Autodesk Inventor part; units mm, degrees
ref_plane "YZ Plane" through (0, 0, 0) normal (1, 0, 0) x (0, 1, 0)
ref_plane "XZ Plane" through (0, 0, 0) normal (0, 1, 0) x (-1, 0, 0)
ref_plane "XY Plane" through (0, 0, 0) normal (0, 0, 1) x (1, 0, 0)
sketch "Sketch1" plane through (0, 0, 0) normal (0, 1, 0) x (-1, 0, 0)
  circle A0 centre (0, 0) radius 30
  dimension "d0" = 60
extrude "Extrusion1" add sketch "Sketch1" along normal blind 10
sketch "Sketch2" plane through (0, 10, 0) normal (0, 1, 0) x (1, 0, 0)
  circle A0 centre (0, 0) radius 5
  dimension "d3" = 10
extrude "Extrusion2" cut sketch "Sketch2" against normal through all
sketch "Sketch3" plane through (0, 10, 0) normal (0, 1, 0) x (1, 0, 0)
  circle A0 centre (0, 0) radius 25
  dimension "d6" = 50
extrude "Extrusion3" add sketch "Sketch3" along normal blind 20
sketch "Sketch5" plane through (0, 30, 0) normal (0, 1, 0) x (1, 0, 0)
  circle A0 centre (0, 0) radius 30
  dimension "d9" = 60
extrude "Extrusion4" add sketch "Sketch5" along normal blind 10
sketch "Sketch6" plane through (0, 40, 0) normal (0, 1, 0) x (1, 0, 0)
  circle A0 centre (0, 0) radius 5
  dimension "d12" = 10
extrude "Extrusion5" cut sketch "Sketch6" against normal through all
properties part number "pulley"
Check sheet for the modelled part. Datum: model origin and axes. Units: mm. A direction names the side the tool comes from. Give positions to 0.01 mm unless a question says otherwise; leave off trailing zeros. Loops run counter-clockwise (first coordinate to the right, second up) from the corner with the lowest first, then second, coordinate; pieces in that order, holes last. Notation, with made-up numbers: M 78,29 L 135,29 A21 cw 135,53 Z; hole C 51.5,59 d3. An arc over 180 degrees is marked long. Use a Markdown table: item, result. Add a question column.
Q1. Scan lines: line 1 along Z through (x, y) = (0, 24); line 2 along Y through (x, z) = (10.5, 26). Record each from-to range of solid material in increasing order. Write a range as [from, to].
Q2. Sectioned sample at A-A, the plane x = 0. Record the cut outline in (y, z), then the cut area to 3 significant figures.
Q3. Mould release check, pull along Y, two halves, no side actions. Record for faces 3 (the cylindrical face through (23.846, 19.86, 7.509)), 4 (the flat face through (0, 40, 6)), 5 (the flat face through (0, 0, -6)), 6 (the cylindrical face through (-29.97, 34.93, 1.32)): pulls with the +Y half, pulls with the -Y half, needs draft (parallel to the pull), parting line crosses it, or undercut.
Q4. Sectioned sample at D-D, the plane x = 26. Record the cut outline in (y, z).
Q5. Tool access check on faces 1 (the cylindrical face through (-1.08, 20.28, 4.88)), 2 (the flat face through (-7, 30, -25)). Record the directions out of +Z, -Z, +X, -X, +Y, -Y that give a thin tool (end or side, any length) a straight path to the whole face; none if there is none.
Q6. Sectioned sample at B-B, the plane z = 0. Record the cut outline in (x, y), then the cut area to 3 significant figures.
Q7. Sectioned sample at C-C, the plane y = 27. Record the cut outline in (x, z), then the cut area to 3 significant figures.
Q8. Go/stop test with flat-tipped pins: pin 1 (10 mm diameter, centred on y = 29.5, z = 21.5, fed in from +X); pin 2 (4 mm diameter, centred on y = 12.5, z = -9, fed in from +X); pin 3 (12 mm diameter, centred on x = -22, y = 17.5, fed in from +Z). Record where each tip stops, or that it passes through.
Verdict:
| question | item | result |
|---|---|---|
| 1 | line 1 | [-25, -5], [5, 25] |
| 1 | line 2 | [0, 10], [30, 40] |
| 2 | outline | M 0,-30 L 10,-30 L 10,-25 L 30,-25 L 30,-30 L 40,-30 L 40,-5 L 0,-5 Z; M 0,5 L 40,5 L 40,30 L 30,30 L 30,25 L 10,25 L 10,30 L 0,30 Z |
| 2 | area | 1,800 mm^2 |
| 3 | face 3 | undercut |
| 3 | face 4 | pulls with the +Y half |
| 3 | face 5 | pulls with the -Y half |
| 3 | face 6 | needs draft |
| 4 | outline | M 0,-14.97 L 10,-14.97 L 10,14.97 L 0,14.97 Z; M 30,-14.97 L 40,-14.97 L 40,14.97 L 30,14.97 Z |
| 5 | face 1 | +Y, -Y |
| 5 | face 2 | none |
| 6 | outline | M -30,0 L -5,0 L -5,40 L -30,40 L -30,30 L -25,30 L -25,10 L -30,10 Z; M 5,0 L 30,0 L 30,10 L 25,10 L 25,30 L 30,30 L 30,40 L 5,40 Z |
| 6 | area | 1,800 mm^2 |
| 7 | outline | C 0,0 d50; hole C 0,0 d10 |
| 7 | area | 1,880 mm^2 |
| 8 | pin 1 | x = 25.04 |
| 8 | pin 2 | x = 24 |
| 8 | pin 3 | z = 19.21 |
